```python
from build123d import *

# Parameters (mm, degrees)
SKETCH1_W           = 109
SKETCH1_H           = 35
SKETCH1_R           = 2.1
SKETCH1_R_2         = 2.6
SKETCH1_W_2         = 12
SKETCH1_H_2         = 3.42
BOSS_EXTRUDE1_DEPTH = 2
FILLET1_R           = 1.5


with BuildPart() as part:
    # Sketch1 → Boss-Extrude1 (new body)
    with BuildSketch(Plane(origin=(0, 0, 0), x_dir=(0, 0, -1), z_dir=(1, 0, 0))):
        with Locations((54.5, -17.5)):
            Rectangle(SKETCH1_W, SKETCH1_H)
        with Locations((104, -8.5)):
            Circle(SKETCH1_R, mode=Mode.SUBTRACT)
        with Locations(Location((104, -26.5, 0), (0, 0, 180))):
            Circle(SKETCH1_R, mode=Mode.SUBTRACT)
        with Locations((80, -26.5)):
            Circle(SKETCH1_R, mode=Mode.SUBTRACT)
        with Locations(Location((80, -8.5, 0), (0, 0, 180))):
            Circle(SKETCH1_R, mode=Mode.SUBTRACT)
        with Locations((5, -26.5)):
            Circle(SKETCH1_R, mode=Mode.SUBTRACT)
        with Locations(Location((5, -8.5, 0), (0, 0, 180))):
            Circle(SKETCH1_R, mode=Mode.SUBTRACT)
        with Locations(Location((29, -26.5, 0), (0, 0, 180))):
            Circle(SKETCH1_R, mode=Mode.SUBTRACT)
        with Locations((29, -8.5)):
            Circle(SKETCH1_R, mode=Mode.SUBTRACT)
        with Locations((39.5, -18)):
            Circle(SKETCH1_R_2, mode=Mode.SUBTRACT)
        with Locations(Location((69.5, -18, 0), (0, 0, 180))):
            Circle(SKETCH1_R_2, mode=Mode.SUBTRACT)
        with Locations((54.5, -5.79)):
            Rectangle(SKETCH1_W_2, SKETCH1_H_2, mode=Mode.SUBTRACT)
    extrude(amount=BOSS_EXTRUDE1_DEPTH)

    # Fillet1
    fillet1_edges = [part.edges().sort_by_distance(p)[0] for p in [
        (1, 0, 0),
        (1, 0, -109),
        (1, -35, -109),
        (1, -35, 0),
    ]]
    fillet(fillet1_edges, radius=FILLET1_R)


solid = part.part
```
Part model, mm, in its own coordinate system. A direction names the side the tool comes from. Round coordinates to 2 decimals unless told otherwise and drop trailing zeros. Write each loop counter-clockwise with the first axis right and the second up, starting at its lowest first coordinate (ties: lowest second). Pieces come first, ordered by that corner, then holes. Notation, with made-up numbers: M 50,-31.5 L 61,-31.5 A5 cw 61,-26.5 Z; hole C -34.5,88 d3. An arc over 180 degrees is marked long. One line per question, with ' | ' between items.
(1) 3-axis set-ups, long thin cutter, end or side, ignore diameter. For faces 1 (the face through (0, -17, -54)), 2 (the face through (1, -6, -60.5)): which of +Z, -Z, +X, -X, +Y, -Y reach the whole face in a straight line?
Answer key:
face 1: +Z, -Z, -X, +Y, -Y | face 2: +X, -X
(2) Saw through at C-C on y = -26.5. Write the cut outline in (x, z).
Answer key:
outline: M 0,-109 L 2,-109 L 2,-106.1 L 0,-106.1 Z; M 0,-101.9 L 2,-101.9 L 2,-82.1 L 0,-82.1 Z; M 0,-77.9 L 2,-77.9 L 2,-31.1 L 0,-31.1 Z; M 0,-26.9 L 2,-26.9 L 2,-7.1 L 0,-7.1 Z; M 0,-2.9 L 2,-2.9 L 2,0 L 0,0 Z
(3) Saw through at A-A on z = -39.5. Write the cut outline in (x, y), then the cut area to 3 significant figures.
Answer key:
outline: M 0,-35 L 2,-35 L 2,-20.6 L 0,-20.6 Z; M 0,-15.4 L 2,-15.4 L 2,0 L 0,0 Z | area: 59.6 mm^2
(4) Saw through at B-B on x = 1.1. Count the separate pieces of the cut face and the enclosed holes in it, then the cut area to 3 significant figures.
Answer key:
separate pieces: 1 | enclosed holes: 11 | area: 3,620 mm^2
(5) Probe line 1 along Y through (x, z) = (1.5, -80); line 2 along Y through (x, z) = (1.8, -103.5); line 3 along Z through (x, y) = (1.55, -19). List the from-to ranges inside material, lowest first.
Answer key:
line 1: y = -35 to -28.6, -24.4 to -10.6, -6.4 to 0 | line 2: y = -35 to -28.54, -24.46 to -10.54, -6.46 to 0 | line 3: z = -109 to -71.9, -67.1 to -41.9, -37.1 to 0
(6) Saw through at D-D on z = -5. Write the cut outline in (x, y), then the cut area to 3 significant figures.
Answer key:
outline: M 0,-35 L 2,-35 L 2,-28.6 L 0,-28.6 Z; M 0,-24.4 L 2,-24.4 L 2,-10.6 L 0,-10.6 Z; M 0,-6.4 L 2,-6.4 L 2,0 L 0,0 Z | area: 53.2 mm^2
(7) Two-plate mould, pull along Y, no slides. Class faces 3 (the face through (0.986, -7.081, -27.452)), 4 (the face through (1, -18, -109)), 5 (the face through (1, 0, -54)): released by +Y, released by -Y, zero draft, split by the parting line, or undercut.
Answer key:
face 3: undercut | face 4: zero draft | face 5: released by +Y
(8) Pin check, flat tip, straight feed: pin 1 (3.5 mm diameter, centred on y = -8.5, z = -80, fed in from +X). Stop position of the tip, or through.
Answer key:
pin 1: passes through
